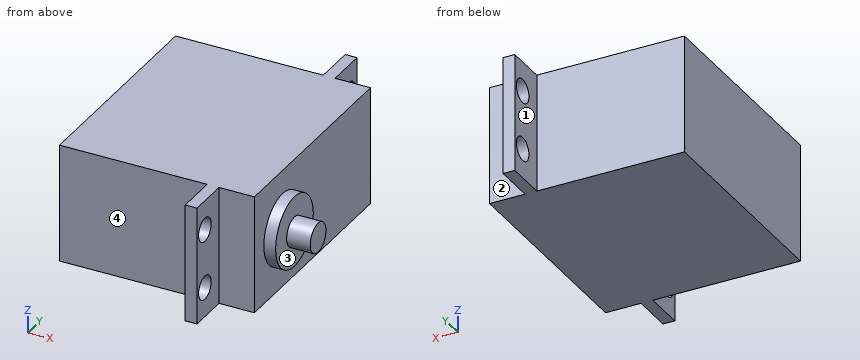
```python
from build123d import *

# Parameters (mm, degrees)
ESQUISSE2_W                   = 33
ESQUISSE2_H                   = 20
BOSS_EXTRU_1_DEPTH            = 18.5
ESQUISSE3_W                   = 2
ESQUISSE3_H                   = 20
BOSS_EXTRU_2_DEPTH            = 7
ESQUISSE4_R                   = 6
BOSS_EXTRU_3_DEPTH            = 2
ESQUISSE5_R                   = 2.5
BOSS_EXTRU_4_DEPTH            = 4
DIAM_TRE_DU_PER_AGE_4_0_4_1_D = 4


with BuildPart() as part:
    # Esquisse2 → Boss.-Extru.1 (new body)
    with BuildSketch(Plane(origin=(0, 0, 0), x_dir=(1, 0, 0), z_dir=(0, 1, 0))):
        with Locations((16.5, 10)):
            Rectangle(ESQUISSE2_W, ESQUISSE2_H)
    boss_extru_1 = extrude(amount=BOSS_EXTRU_1_DEPTH)

    # Esquisse3 → Boss.-Extru.2 (add)
    with BuildSketch(Plane.XZ):
        with Locations((26, -10)):
            Rectangle(ESQUISSE3_W, ESQUISSE3_H)
    boss_extru_2 = extrude(amount=BOSS_EXTRU_2_DEPTH)

    # Symétrie1: Boss.-Extru.1, Boss.-Extru.2 across plane
    add(boss_extru_1.mirror(Plane(origin=(0, 18.5, 0), x_dir=(0, 0, 1), z_dir=(0, -1, 0))))
    add(boss_extru_2.mirror(Plane(origin=(0, 18.5, 0), x_dir=(0, 0, 1), z_dir=(0, -1, 0))))

    # Esquisse4 → Boss.-Extru.3 (add)
    with BuildSketch(Plane(origin=(33, 0, 0), x_dir=(0, 0, -1), z_dir=(1, 0, 0))):
        with Locations(Location((10, 9, 0), (0, 0, 180))):
            Circle(ESQUISSE4_R)
    extrude(amount=BOSS_EXTRU_3_DEPTH)

    # Esquisse5 → Boss.-Extru.4 (add)
    with BuildSketch(Plane(origin=(35, 0, 0), x_dir=(0, 0, -1), z_dir=(1, 0, 0))):
        with Locations((10, 9)):
            Circle(ESQUISSE5_R)
    extrude(amount=BOSS_EXTRU_4_DEPTH)

    # Diamètre du perçage Ø4.0 (4)1 (through all)
    with Locations(Plane(origin=(27, 0, 0), x_dir=(0, 0, -1), z_dir=(1, 0, 0))):
        with Locations((15, 41.5), (5, 41.5), (15, -4.5), (5, -4.5)):
            Hole(DIAM_TRE_DU_PER_AGE_4_0_4_1_D / 2)


solid = part.part
```
Model file for the job. Use its own axes, mm. Face numbers are marked on the shaded views. A direction names the side the tool comes from. Give positions to 0.01 mm unless a question says otherwise; leave off trailing zeros. Write each loop counter-clockwise with the first axis right and the second up, starting at its lowest first coordinate (ties: lowest second). Pieces come first, ordered by that corner, then holes. Notation, with made-up numbers: (65.5, -11.75) - (85.5, -11.75) arc R25 ccw to (85.5, 4.25) - close; hole circle Ø2 at (4, -35). An arc over 180 degrees is marked (long way). One line per question, with ' | ' between items. Start each with the question number.
(1) Slice it at B-B on y = 9. Write the cut outline in (x, z), plus the area to 3 significant figures.
(2) Slice it at D-D on z = -10. Write the cut outline in (x, y).
(3) Pin check, flat tips, straight feed: P1, Ø6, axis at y = 37.5, z = -11, coming from the +X side; P2, Ø5, axis at x = 31, z = -13.5, coming from the +Y side; P3, Ø6.5, axis at y = -4.5, z = -15, coming from the -X side. Stop position of each tip, or through.
(4) Slice it at C-C on z = -15. Write the cut outline in (x, y), plus the area to 3 significant figures.
(5) Slice it at A-A on y = -4.5. Write the cut outline in (x, z), plus the area to 3 significant figures.
(6) Wall check: line 1 along Y through (x, z) = (26, -15); line 2 along Z through (x, y) = (26, 41); line 3 along X through (y, z) = (21, -14). Give the ranges that are in metal, low to high. Write a range as from..to.
(7) 3-axis set-ups, long thin cutter, end or side, ignore diameter. For the marked faces 1, 2, 3 and 4: which of +Z, -Z, +X, -X, +Y, -Y reach the whole face in a straight line?
Results below:
1) outline: (0, -20) - (33, -20) - (33, -16) - (35, -16) - (35, -12.5) - (39, -12.5) - (39, -7.5) - (35, -7.5) - (35, -4) - (33, -4) - (33, 0) - (0, 0) - close | area: 704 mm^2
2) outline: (0, 0) - (25, 0) - (25, -7) - (27, -7) - (27, 0) - (33, 0) - (33, 3) - (35, 3) - (35, 6.5) - (39, 6.5) - (39, 11.5) - (35, 11.5) - (35, 15) - (33, 15) - (33, 37) - (27, 37) - (27, 44) - (25, 44) - (25, 37) - (0, 37) - close
3) P1: x = 33 | P2: y = 37 | P3: x = 25
4) outline: (0, 0) - (25, 0) - (25, -2.5) - (27, -2.5) - (27, 0) - (33, 0) - (33, 5.68) - (35, 5.68) - (35, 12.32) - (33, 12.32) - (33, 37) - (27, 37) - (27, 39.5) - (25, 39.5) - (25, 37) - (0, 37) - close; (25, -7) - (27, -7) - (27, -6.5) - (25, -6.5) - close; (25, 43.5) - (27, 43.5) - (27, 44) - (25, 44) - close | area: 1,250 mm^2
5) outline: (25, -20) - (27, -20) - (27, -17) - (25, -17) - close; (25, -13) - (27, -13) - (27, -7) - (25, -7) - close; (25, -3) - (27, -3) - (27, 0) - (25, 0) - close | area: 24.0 mm^2
6) line 1: -7..-6.5, -2.5..39.5, 43.5..44 | line 2: -20..-16.94, -13.06..-6.94, -3.06..0 | line 3: 0..33
7) face 1: +Z, -Z, -X, +Y | face 2: +Z, -Z, +X, +Y | face 3: +X | face 4: +Z, -Z, -X, -Y
